from build123d import *

# Parameters (mm, degrees)
F1_DEPTH = 265.43
F3_DEPTH = 25.4
F5_DEPTH = 2.54


with BuildPart() as f1:
    # F0 (on Front) → F1 (new body)
    with BuildSketch(Plane.XZ):
        Polygon((-2.54, 0), (0, 0), (0, 18.415), (-25.4, 18.415), (-25.4, 15.875), (-2.54, 15.875), (-2.54, 15.24), (-5.08, 15.24), (-5.08, 12.446), (-3.81, 12.446), (-3.81, 13.97), (-2.54, 13.97), (-2.54, 7.62), (-3.81, 7.62), (-3.81, 9.144), (-5.08, 9.144), (-5.08, 6.35), (-2.54, 6.35), align=None)
    extrude(amount=F1_DEPTH)

    # F2 (on face) → F3 (cut)
    with BuildSketch(Plane.YZ):
        Polygon((-247.015, 0), (-265.43, 18.415), (-265.43, 0), align=None)
        Polygon((0, 0), (0, 18.415), (-18.415, 0), align=None)
    extrude(amount=-F3_DEPTH, mode=Mode.SUBTRACT)

    # F4 (on face) → F5 (cut)
    with BuildSketch(Plane.XY.offset(18.415)):
        with BuildLine():
            Line((-6.985, -240.3475), (-20.32, -240.3475))
            ThreePointArc((-20.32, -240.3475), (-21.9075, -241.935), (-20.32, -243.5225))
            Line((-20.32, -243.5225), (-6.985, -243.5225))
            ThreePointArc((-6.985, -243.5225), (-5.3975, -241.935), (-6.985, -240.3475))
        make_face()
        with BuildLine():
            ThreePointArc((-20.32, -21.9075), (-21.9075, -23.495), (-20.32, -25.0825))
            Line((-20.32, -25.0825), (-6.985, -25.0825))
            ThreePointArc((-6.985, -25.0825), (-5.3975, -23.495), (-6.985, -21.9075))
            Line((-6.985, -21.9075), (-20.32, -21.9075))
        make_face()
    extrude(amount=-F5_DEPTH, mode=Mode.SUBTRACT)


solid = f1.part
Model file for the job. Use its own axes, mm. Give positions to 0.01 mm unless a question says otherwise; leave off trailing zeros. Order: outer loops, then holes, each group sorted by start corner. A loop starts at its lowest first (then second) coordinate and runs counter-clockwise, first axis right, second up. Notation, with made-up numbers: M -0.75,43.5 L 35.25,43.5 A18 cw 35.25,62.5 Z; hole C 82,60 d1. An arc over 180 degrees is marked long. Put each result on its own line as item: value. Start each with the question number.
(1) Drill centre lines: L1, parallel to Z at x = -4.75, y = -121.5 (3 decimals); L2, parallel to Z at x = -10.5, y = -234.5 (3 decimals); L3, parallel to X at y = -85, z = 2. Where is each one in solid material? Low to high. Write a range as [from, to].
(2) Pull direction Z, two halves, no side cores. Call faces 1 (the face through (-2.54, -131, 11)), 2 (the face through (-2.54, -131, 3)), 3 (the face through (-7.937, -2.344, 16.071)), 4 (the face through (-13, -131, 18.415)): released by +Z, released by -Z, zero draft, split by the parting line, or undercut.
(3) Pin check, flat tips, straight feed: pin 1 Ø2 at (y, z) = (-230, 2.5) entering from -X; pin 2 Ø3 at (y, z) = (-123, 13.5) entering from -X; pin 3 Ø6 at (x, y) = (-14, -28.5) entering from -Z (3 decimals). Stop position of each tip, or through.
(4) Band-saw the part on A-A on y = -40.5. Give the cut face in (x, z) (3 decimals).
Results below:
1. L1: z = [6.35, 9.144], [12.446, 15.24], [15.875, 18.415]
1. L2: z = [15.875, 18.415]
1. L3: x = [-2.54, 0]
2. face 1: undercut
2. face 2: zero draft
2. face 3: released by -Z
2. face 4: released by +Z
3. pin 1: stops at x = -2.54
3. pin 2: stops at x = -5.08
3. pin 3: stops at z = 15.875
4. outline: M -25.4,15.875 L -2.54,15.875 L -2.54,15.24 L -5.08,15.24 L -5.08,12.446 L -3.81,12.446 L -3.81,13.97 L -2.54,13.97 L -2.54,7.62 L -3.81,7.62 L -3.81,9.144 L -5.08,9.144 L -5.08,6.35 L -2.54,6.35 L -2.54,0 L 0,0 L 0,18.415 L -25.4,18.415 Z
